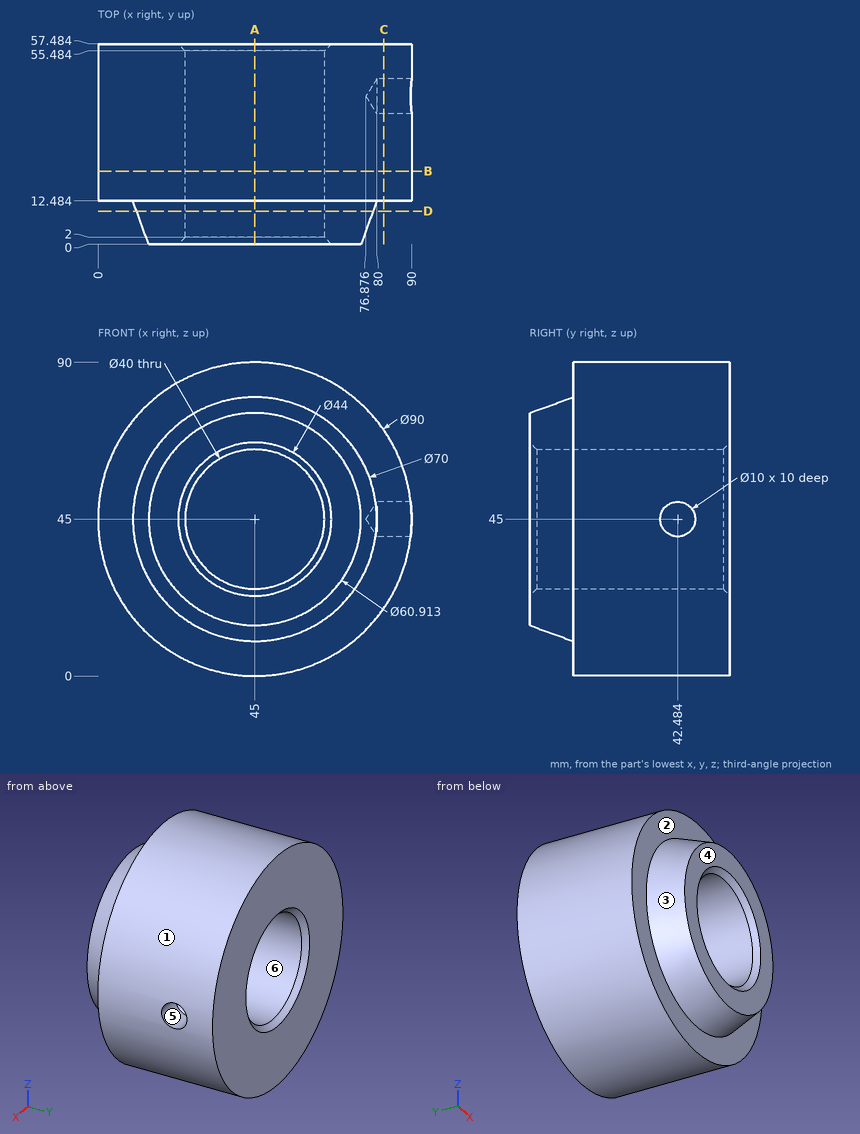
Could you check a few things on this drawing? It's one solid part, dimensions in mm from its lowest x, y, z. A direction names the side the tool comes from. Coordinates: 2 decimals unless noted, no trailing zeros. Order: outer loops, then holes, each group sorted by start corner. A loop starts at its lowest first (then second) coordinate and runs counter-clockwise, first axis right, second up.
1. I'm going to push flat-ended pins straight in: pin 1 (1 mm diameter, centred on x = 28.5, z = 55.5, fed in from +Y); pin 2 (10 mm diameter, centred on y = 39, z = 25, fed in from +X); pin 3 (5 mm diameter, centred on x = 18, y = 21, fed in from +Z) (1 decimal). Where does each tip first touch, or does it pass through?
2. If we section it at C-C (x = 82): Please give me the cut outline in (y, z).
3. I need wall thicknesses on line 1 (Y direction, x = 37, z = 79.5); line 2 (Z direction, x = 45, y = 24); line 3 (X direction, y = 41.5, z = 55.5). Which ranges of each line are inside material? Lowest first, please.
4. If we section it at A-A (x = 45): Please give me the cut outline in (y, z), then the cut area to 3 significant figures.
5. If we section it at B-B (y = 21): Please give me the cut outline in (x, z), then the cut area to 4 significant figures.
6. Thinking about a two-plate mould opening in Z: for the marked faces 3, 4, 5 and 6, which applies, +Z half, -Z half, draft (parallel to the pull), parting line (faces both ways), or undercut?
7. If we section it at D-D (y = 9.5): Please give me the cut outline in (x, z), then the cut area to 3 significant figures.
8. For the marked faces 1 and 2, which set-ups out of +Z, -Z, +X, -X, +Y, -Y let a thin tool reach every point of the face, with its end or its side?
Entries:
1. pin 1: stops at y = 55.54
1. pin 2: stops at x = 87.43
1. pin 3: stops at z = 82.7
2. outline: (12.48, 19.39) - (57.48, 19.39) - (57.48, 70.61) - (12.48, 70.61) - close; hole circle Ø10 at (42.48, 45)
3. line 1: y = 12.48 to 57.48
3. line 2: z = 0 to 25, 65 to 90
3. line 3: x = 1.24 to 27.98, 62.02 to 88.76
4. outline: (0, 14.54) - (12.48, 10) - (12.48, 0) - (57.48, 0) - (57.48, 23) - (55.48, 25) - (2, 25) - (0, 23) - close; (0, 67) - (2, 65) - (55.48, 65) - (57.48, 67) - (57.48, 90) - (12.48, 90) - (12.48, 80) - (0, 75.46) - close
4. area: 2,560 mm2
5. outline: circle Ø90 at (45, 45); hole circle Ø40 at (45, 45)
5. area: 5,105 mm2
6. face 3: parting line
6. face 4: draft
6. face 5: undercut
6. face 6: undercut
7. outline: circle Ø67.83 at (45, 45); hole circle Ø40 at (45, 45)
7. area: 2,360 mm2
8. face 1: +Y, -Y
8. face 2: -Y
